Input: part model. Units: mm. Frame: model coordinates. Face numbers are marked on the shaded views. A direction names the side the tool comes from. Coordinates: 2 decimals unless noted, no trailing zeros. Order: outer loops, then holes, each group sorted by start corner. A loop starts at its lowest first (then second) coordinate and runs counter-clockwise, first axis right, second up.
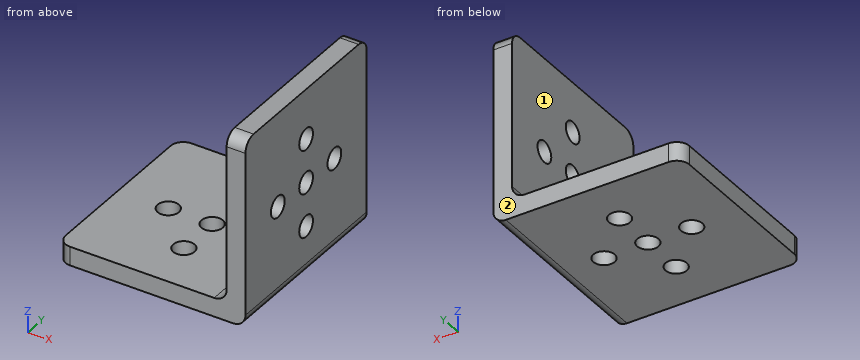
from build123d import *

# Parameters (mm, degrees)
SKETCH1_W                      = 27
SKETCH1_H                      = 30
BOSS_EXTRUDE1_DEPTH            = 3
SKETCH1_3_W                    = 3
SKETCH1_3_H                    = 30
BOSS_EXTRUDE2_DEPTH            = 30
M3_CLEARANCE_HOLE1_D           = 3.4
M3_CLEARANCE_HOLE1_ON_FACE_2_D = 3.4
M3_CLEARANCE_HOLE2_D           = 3.4
FILLET1_R                      = 2
FILLET2_R                      = 2


with BuildPart() as part:
    # Sketch1 → Boss-Extrude1 (new body)
    with BuildSketch(Plane.XY):
        with Locations((-1.5, 0)):
            Rectangle(SKETCH1_W, SKETCH1_H)
    extrude(amount=BOSS_EXTRUDE1_DEPTH)

    # Sketch1<3> → Boss-Extrude2 (add)
    with BuildSketch(Plane.XY):
        with Locations((13.5, 0)):
            Rectangle(SKETCH1_3_W, SKETCH1_3_H)
    extrude(amount=BOSS_EXTRUDE2_DEPTH)

    # M3 Clearance Hole1 (through all)
    with Locations(Plane(origin=(0, 7, 3), x_dir=(1, 0, 0), z_dir=(0, 0, 1))):
        with Locations((0, 0), (-7, -7), (7, -7), (0, -14), (0, -7)):
            Hole(M3_CLEARANCE_HOLE1_D / 2)

    # M3 Clearance Hole1 on face 2 (through all)
    with Locations(Plane(origin=(0, 0, 0), x_dir=(-1, 0, 0), z_dir=(0, 0, -1))):
        with Locations((0, 0)):
            Hole(M3_CLEARANCE_HOLE1_ON_FACE_2_D / 2)

    # M3 Clearance Hole2 (through all)
    with Locations(Plane(origin=(15, 7, 15), x_dir=(0, 1, 0), z_dir=(1, 0, 0))):
        with Locations((0, 0), (-7, 7), (-7, 0), (-7, -7), (-14, 0)):
            Hole(M3_CLEARANCE_HOLE2_D / 2)

    # Fillet1
    fillet1_edges = [part.edges().sort_by_distance(p)[0] for p in [
        (15, 0, 0),
        (12, 0, 3),
    ]]
    fillet(fillet1_edges, radius=FILLET1_R)

    # Fillet2
    fillet2_edges = [part.edges().sort_by_distance(p)[0] for p in [
        (13.5, 15, 30),
        (13.5, -15, 30),
        (-15, -15, 1.5),
        (-15, 15, 1.5),
    ]]
    fillet(fillet2_edges, radius=FILLET2_R)


solid = part.part
Item 1: Cut plane D-D on y = 0. Count the separate pieces of the cut face and the enclosed holes in it, then the cut area to 3 significant figures.
Response values:
separate pieces: 7
enclosed holes: 0
area: 110 mm2
Item 2: Cut plane B-B on z = 22. Return loops of the section in (x, y), then the cut area to 3 significant figures.
Response values:
outline: (12, -15) - (15, -15) - (15, -1.7) - (12, -1.7) - close; (12, 1.7) - (15, 1.7) - (15, 15) - (12, 15) - close
area: 79.8 mm2
Item 3: Cut plane A-A on x = 0. Return loops of the section in (y, z), then the cut area to 3 significant figures.
Response values:
outline: (-15, 0) - (-8.7, 0) - (-8.7, 3) - (-15, 3) - close; (-5.3, 0) - (-1.7, 0) - (-1.7, 3) - (-5.3, 3) - close; (1.7, 0) - (5.3, 0) - (5.3, 3) - (1.7, 3) - close; (8.7, 0) - (15, 0) - (15, 3) - (8.7, 3) - close
area: 59.4 mm2
Item 4: Cut plane C-C on z = 15. Return loops of the section in (x, y).
Response values:
outline: (12, -15) - (15, -15) - (15, -8.7) - (12, -8.7) - close; (12, -5.3) - (15, -5.3) - (15, -1.7) - (12, -1.7) - close; (12, 1.7) - (15, 1.7) - (15, 5.3) - (12, 5.3) - close; (12, 8.7) - (15, 8.7) - (15, 15) - (12, 15) - close
Item 5: Ray query, probe 1 along Y at (x, z) = (0, 2.2); probe 2 along Y at (x, z) = (7, 1.45); probe 3 along X at (y, z) = (-1.5, 24). Return the intervals inside material, ascending.
Response values:
probe 1: y = -15 to -8.7, -5.3 to -1.7, 1.7 to 5.3, 8.7 to 15
probe 2: y = -15 to -1.7, 1.7 to 15
probe 3: x = 12 to 15
Item 6: Access query for the marked faces 1 and 2. Directions: +Z, -Z, +X, -X, +Y, -Y. A direction counts if a zero-diameter tool reaches every point of the face in a straight line with its end or side. Return the directions, or none.
Response values:
face 1: +Z, -X, +Y, -Y
face 2: +Z, -Z, +X, -X, +Y
Item 7: Pin query (flat end, axial travel): pin 1 Ø3 at (y, z) = (11.5, 6.5) entering from -X; pin 2 Ø5.5 at (x, y) = (0, -7) entering from -Z; pin 3 Ø5.5 at (x, y) = (7, 0) entering from +Z. Return the tip coordinate at first contact, or that it passes through.
Response values:
pin 1: stops at x = 12
pin 2: stops at z = 0
pin 3: stops at z = 3
